Autodesk Inventor part; units mm, degrees
ref_plane "YZ Plane" through (0, 0, 0) normal (1, 0, 0) x (0, 1, 0)
ref_plane "XZ Plane" through (0, 0, 0) normal (0, 1, 0) x (-1, 0, 0)
ref_plane "XY Plane" through (0, 0, 0) normal (0, 0, 1) x (1, 0, 0)
sketch "Sketch1" plane through (0, 0, 0) normal (0, 0, 1) x (1, 0, 0)
  line L0 (-22, 0) -> (22, 0) construction
  line L1 (-22, -40) -> (22, -40)
  line L2 (22, 40) -> (-22, 40)
  arc A0 (-22, 40) -> (-22, -40) centre (-22, 0) ccw
  arc A1 (22, -40) -> (22, 40) centre (22, 0) ccw
  line L3 (-22, 0) -> (22, 0) construction
  line L4 (-22, -16) -> (22, -16)
  line L5 (22, 16) -> (-22, 16)
  arc A2 (-22, 16) -> (-22, -16) centre (-22, 0) ccw
  arc A3 (22, -16) -> (22, 16) centre (22, 0) ccw
  line L6 (22, 10) -> (-22, 10)
  arc A4 (-22, 10) -> (-22, -10) centre (-22, 0) ccw
  line L7 (-22, -10) -> (22, -10)
  arc A5 (22, -10) -> (22, 10) centre (22, 0) ccw
  point P0 (0, 0)
  point P1 (0, 0)
  point P2 (62, 0)
  point P3 (-62, 0)
  point P4 (0, 0)
  point P5 (38, 0)
  point P6 (-38, 0)
  point P7 (-48, 0)
  point P8 (-22, -26)
  dimension "d1" = 124
  dimension "d2" = 76
  dimension "d3" = 80
  dimension "d4" = 16
  dimension "d5" = 10
  dimension "d6" = 26
  dimension "d7" = 26
extrude "Extrusion1" add sketch "Sketch1" along normal blind 10 contours A0 L2 A1 L1 | A2 L5 A3 L4 | A5 L7 A4 L6
extrude "Extrusion2" add sketch "Sketch1" along normal blind 32 contours A2 L5 A3 L4 | A5 L7 A4 L6
extrude "Extrusion3" cut sketch "Sketch1" against normal blind 10 from surface at 32 contours A5 L7 A4 L6
hole "Hole1" at (-22, -26, 0) at (-48, 0, 0) direction (0, 0, 1) diameter 6 depth 10
sketch "Sketch2" plane through (0, 0, 10) normal (0, 0, 1) x (1, 0, 0)
  circle A0 centre (-48, 0) radius 3
  circle A1 centre (-22, -26) radius 3
  point P0 (0, 0)
hole "Hole2" at (-48, 0, 10) at (-22, -26, 10) direction (0, 0, -1) diameter 13 depth 2
hole "Hole3" at (-22, 0, 0) direction (0, 0, 1) diameter 10 depth 22
mirror "Mirror1" about plane through (0, 0, 0) normal (1, 0, 0) of "Hole2", "Hole3", "Hole1"
mirror "Mirror2" about plane through (0, 0, 0) normal (0, 1, 0) of "Hole2", "Hole1", "Hole3", "Mirror1"
fillet "Fillet1" radius 2 8 edges at (62, 0, 10) (0, 40, 10) (-62, 0, 10) (0, -40, 10) (0, -16, 10) (-38, 0, 10) (0, 16, 10) (38, 0, 10)
move or copy body "Rotate1" bodies to move or copy 1 copy no rotation origin (0, 0, 0) rotation axis (1, 0, 0) rotation angle -90
properties part number "b2"
Can you work these out from the model? Positions are in its coordinate system, mm. A direction names the side the tool comes from. Round coordinates to 2 decimals unless told otherwise and drop trailing zeros. Loops run counter-clockwise (first coordinate to the right, second up) from the corner with the lowest first, then second, coordinate; pieces in that order, holes last. Notation, with made-up numbers: (62, 1.5) - (105, 1.5) arc R30 ccw to (105, 26.5) - close; hole circle Ø2 at (-6, 5.25). An arc over 180 degrees is marked (long way). Use CSV: the item, a comma, the result in double quotes. Start each with the question number.
1) We'd pull the mould along X, two halves only. Please class faces 1 (the cylindrical face through (45, 4, 0)), 2 (the flat face through (0, 22, 16)), 3 (the cylindrical face through (-38, 22, 0)): released by +X, released by -X, zero draft, split by the parting line, or undercut.
2) Please list where these lines run through material, in increasing order: probe 1 along X at (y, z) = (2.5, 26); probe 2 along X at (y, z) = (9.45, 0); probe 3 along X at (y, z) = (9.35, 0). Write a range as [from, to].
3) For pin 1 Ø6 at (x, y) = (-9.5, 24.5) entering from -Z; pin 2 Ø6.5 at (x, z) = (21, 24.5) entering from +Y; pin 3 Ø6 at (x, y) = (-32.5, 18.5) entering from -Z, each with a flat end and sliding along its axis, tell me the tip position at first contact or that it passes through.
4) If we section it at A-A on y = 25.5: Write out the boundary of the cut face in (x, z), plus the area to 3 significant figures.
5) If we section it at C-C on z = -26: Count the separate pieces of the cut face and the enclosed holes in it, plus the area to 3 significant figures.
6) If we section it at B-B on x = 6: Write out the boundary of the cut face in (y, z), plus the area to 3 significant figures.
7) For faces 4 (the cylindrical face through (-23.8, 4.1, -28.4)), 5 (the cylindrical face through (-17.607, 8.986, -21.209)), which set-ups out of +Z, -Z, +X, -X, +Y, -Y let a thin tool reach every point of the face, with its end or its side?
Geometry results:
1,face 1,"undercut"
1,face 2,"zero draft"
1,face 3,"released by -X"
2,probe 1,"x = [-52.4, -25], [-19, 19], [25, 52.4]"
2,probe 2,"x = [-61.38, -54.5], [-41.5, -27], [-17, 17], [27, 41.5], [54.5, 61.38]"
2,probe 3,"x = [-61.48, -54.5], [-41.5, -27], [-17, 17], [27, 41.5], [54.5, 61.48]"
3,pin 1,"stops at z = -16"
3,pin 2,"stops at y = 8"
3,pin 3,"stops at z = -14.13"
4,outline,"(-22, -16) - (22, -16) arc R16 ccw to (22, 16) - (-22, 16) arc R16 ccw to start; hole (-22, -10) - (22, -10) arc R10 ccw to (22, 10) - (-22, 10) arc R10 ccw to start"
4,area,"1,020 mm2"
5,separate pieces,"3"
5,enclosed holes,"0"
5,area,"898 mm2"
6,outline,"(0, -40) - (8, -40) arc R2 ccw to (10, -38) - (10, -18) arc R2 cw to (12, -16) - (32, -16) - (32, -10) - (22, -10) - (22, 10) - (32, 10) - (32, 16) - (12, 16) arc R2 cw to (10, 18) - (10, 38) arc R2 ccw to (8, 40) - (0, 40) - close"
6,area,"1,300 mm2"
7,face 4,"+Y, -Y"
7,face 5,"+Y"
